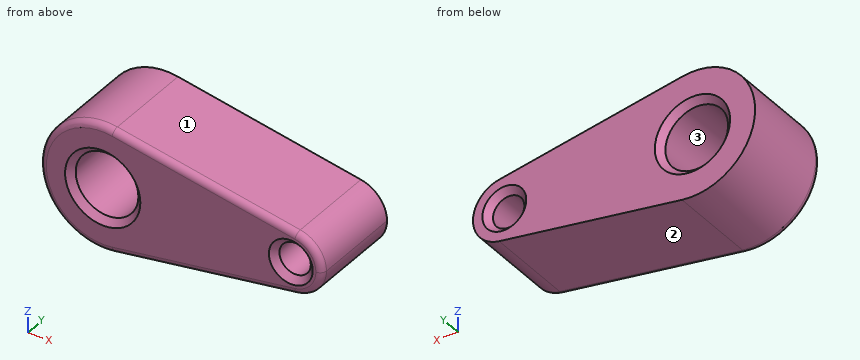
from build123d import *

# Parameters (mm, degrees)
F0_R     = 25.4
F0_R_2   = 12.7
F1_DEPTH = 76.2
F2_SIZE  = 5.08
F3_SIZE  = 5.08
F4_R     = 5.08


with BuildPart() as f1:
    # F0 (on Front) → F1 (new body)
    with BuildSketch(Plane.XZ):
        with BuildLine():
            ThreePointArc((8.466667, -50.089475), (38.799141, -32.791259), (50.8, 0))
            ThreePointArc((50.8, 0), (38.799141, 32.791259), (8.466667, 50.089475))
            ThreePointArc((8.466667, 50.089475), (-50.8, 0), (8.466667, -50.089475))
        make_face()
        Circle(F0_R, mode=Mode.SUBTRACT)
        with BuildLine():
            ThreePointArc((8.466667, 50.089475), (38.799141, 32.791259), (50.8, 0))
            ThreePointArc((50.8, 0), (38.799141, -32.791259), (8.466667, -50.089475))
            Line((8.466667, -50.089475), (156.633333, -25.044738))
            ThreePointArc((156.633333, -25.044738), (127, 0), (156.633333, 25.044738))
            Line((156.633333, 25.044738), (8.466667, 50.089475))
        make_face()
        with BuildLine():
            ThreePointArc((177.8, 0), (171.79957, 16.395629), (156.633333, 25.044738))
            ThreePointArc((156.633333, 25.044738), (127, 0), (156.633333, -25.044738))
            ThreePointArc((156.633333, -25.044738), (171.79957, -16.395629), (177.8, 0))
        make_face()
        with Locations((152.4, 0)):
            Circle(F0_R_2, mode=Mode.SUBTRACT)
    extrude(amount=-F1_DEPTH)

    # F2
    f2_edges = [f1.edges().sort_by_distance(p)[0] for p in [
        (-25.4, 0, 0),
        (-25.4, 76.2, 0),
    ]]
    chamfer(f2_edges, length=F2_SIZE)

    # F3
    f3_edges = [f1.edges().sort_by_distance(p)[0] for p in [
        (139.7, 76.2, 0),
        (139.7, 0, 0),
    ]]
    chamfer(f3_edges, length=F3_SIZE)

    # F4
    f4_edges = [f1.edges().sort_by_distance(p)[0] for p in [
        (82.55, 0, -37.567107),
    ]]
    fillet(f4_edges, radius=F4_R)


solid = f1.part
The model under review builds one solid part; all positions refer to its coordinate system, in mm. Face numbers are marked on the shaded views. Round coordinates to 2 decimals unless told otherwise and drop trailing zeros. Write each loop counter-clockwise with the first axis right and the second up, starting at its lowest first coordinate (ties: lowest second). Pieces come first, ordered by that corner, then holes. Notation, with made-up numbers: M -30.5,30.5 L 12.5,30.5 A25 cw 12.5,48.5 Z; hole C 14,20.5 d4. An arc over 180 degrees is marked long. Use a Markdown table: item, result. Add a question column.
Q1. We need section B-B, the plane z = 3. Count the separate pieces of the cut face and the enclosed holes in it, plus the area to 3 significant figures.
Q2. Insertion check: pin 1 (4 mm diameter, centred on y = 44, z = 29.5, fed in from -X); pin 2 (2 mm diameter, centred on y = 18, z = -14.5, fed in from -X); pin 3 (1.5 mm diameter, centred on x = 149.5, y = 19, fed in from -Z). Each pin has a flat end and moves straight along its axis. Give the tip position at first contact, or say it passes through.
Q3. To check wall thickness, follow line 1 (Z direction, x = 0, y = 24); line 2 (X direction, y = 64.5, z = -3); line 3 (Z direction, x = -8, y = 4). State the ranges of each line that lie inside material, in increasing order.
Q4. The part is to be moulded in two halves that separate along Z. For the marked faces 1, 2 and 3, say which applies: pulls with the +Z half, pulls with the -Z half, needs draft (parallel to the pull), parting line crosses it, or undercut.
Q5. We need section A-A, the plane y = 24. State the section outline as (x, z) points, plus the area to 3 significant figures.
Findings below:
| question | item | result |
|---|---|---|
| 1 | separate pieces | 3 |
| 1 | enclosed holes | 0 |
| 1 | area | 11,600 mm² |
| 2 | pin 1 | stops at x = -42.71 |
| 2 | pin 2 | stops at x = -48.97 |
| 2 | pin 3 | stops at z = -26.38 |
| 3 | line 1 | z = -50.8 to -25.4, 25.4 to 50.8 |
| 3 | line 2 | x = -50.71 to -25.22, 25.22 to 140.06, 164.74 to 177.62 |
| 3 | line 3 | z = -50.05 to -25.24, 25.24 to 50.05 |
| 4 | face 1 | pulls with the +Z half |
| 4 | face 2 | pulls with the -Z half |
| 4 | face 3 | undercut |
| 5 | outline | M 8.47,-50.09 L 156.63,-25.04 A25.4 ccw 177.8,0 A25.4 ccw 156.63,25.04 L 8.47,50.09 A50.8 ccw long Z; hole C 0,0 d50.8; hole C 152.4,0 d25.4 |
| 5 | area | 14,300 mm² |
